```python
from build123d import *

# Parameters (mm, degrees)
SKETCH1_R           = 0.655
BOSS_EXTRUDE1_DEPTH = 16
CUT_EXTRUDE1_START  = -1.25
CUT_EXTRUDE1_DEPTH  = 1.25
SKETCH3_W           = 0.6
SKETCH3_H           = 0.3


with BuildPart() as part:
    # Sketch1 → Boss-Extrude1 (new body)
    with BuildSketch(Plane(origin=(0, 0, 0), x_dir=(1, 0, 0), z_dir=(0, 1, 0))):
        with Locations(Location((0, 0, 0), (0, 0, 270))):
            Circle(SKETCH1_R)
    extrude(amount=BOSS_EXTRUDE1_DEPTH)

    # Sketch2 → Cut-Extrude1 (cut)
    with BuildSketch(Plane(origin=(0, 16, 0), x_dir=(1, 0, 0), z_dir=(0, 1, 0)).offset(CUT_EXTRUDE1_START)):
        with BuildLine():
            Line((0, -0.655), (0, 0.655))
            ThreePointArc((0, 0.655), (0.655, 0), (0, -0.655))
        make_face()
    extrude(amount=CUT_EXTRUDE1_DEPTH, mode=Mode.SUBTRACT)

    # Sketch3 → Revolve1 (revolve)
    with BuildSketch(Plane.XY, mode=Mode.PRIVATE) as revolve1_sk:
        with Locations((0.655, 12)):
            Rectangle(SKETCH3_W, SKETCH3_H)
        with Locations((0.655, 10.7)):
            Rectangle(SKETCH3_W, SKETCH3_H)
    revolve(revolve1_sk.sketch.rotate(Axis((0, 16, 0), (0, -1, 0)), 90), axis=Axis((0, 16, 0), (0, -1, 0)))


solid = part.part
```
The listing builds one solid part. Answer for the finished solid, in the listing's coordinates (mm). A direction names the side the tool comes from. Round coordinates to 2 decimals unless told otherwise and drop trailing zeros. Order: outer loops, then holes, each group sorted by start corner. A loop starts at its lowest first (then second) coordinate and runs counter-clockwise, first axis right, second up. Notation, with made-up numbers: (-21, 27) -> (12, 27) arc R17 ccw to (12, 44) -> close; hole circle Ø2 at (89.5, -4.75). An arc over 180 degrees is marked (long way). Answer as CSV lines item,"result".
Q1. For a pull along Y with two mould halves and no side action, classify faces 1 (the flat face through (0, 0, 0)), 2 (the cylindrical face through (0.65, 11.34, -0.09)), 3 (the cylindrical face through (0.93, 10.7, -0.21)) as +Y half, -Y half, draft (parallel to the pull), parting line (faces both ways), or undercut.
Computed values:
face 1,"-Y half"
face 2,"undercut"
face 3,"draft"
Q2. A cutting plane is placed at C-C on y = 15. Determine the outline of the cut face in (x, z) (3 decimals).
Computed values:
outline,"(0, -0.655) -> (0, 0.655) arc R0.655 ccw to start"
Q3. A cutting plane is placed at B-B on y = 6.75. Determine the outline of the cut face in (x, z) (3 decimals).
Computed values:
outline,"circle Ø1.31 at (0, 0)"
Q4. A cutting plane is placed at A-A on z = 0. Determine the outline of the cut face in (x, y) (3 decimals).
Computed values:
outline,"(-0.955, 10.55) -> (-0.655, 10.55) -> (-0.655, 0) -> (0.655, 0) -> (0.655, 10.55) -> (0.955, 10.55) -> (0.955, 10.85) -> (0.655, 10.85) -> (0.655, 11.85) -> (0.955, 11.85) -> (0.955, 12.15) -> (0.655, 12.15) -> (0.655, 14.75) -> (0, 14.75) -> (0, 16) -> (-0.655, 16) -> (-0.655, 12.15) -> (-0.955, 12.15) -> (-0.955, 11.85) -> (-0.655, 11.85) -> (-0.655, 10.85) -> (-0.955, 10.85) -> close"
Q5. Given pin 1 (0.6 mm diameter, centred on y = 15, z = 0, fed in from +X) (3 decimals), flat-ended and moving along its own axis, determine where the tip first touches the part or whether it passes through.
Computed values:
pin 1,"stops at x = 0.655"
Q6. Consider line 1 (Y direction, x = -0.8, z = -0.3); line 2 (Z direction, x = 0.05, y = 1.25); line 3 (Y direction, x = 0.5, z = 0.3). Determine where each line is inside the solid, lowest interval first. Write a range as from..to.
Computed values:
line 1,"y = 10.55..10.85, 11.85..12.15"
line 2,"z = -0.65..0.65"
line 3,"y = 0..14.75"
Q7. Which of the six approach directions +Z, -Z, +X, -X, +Y, -Y give full straight-line access (tool end or side, diameter ignored) to faces 4 (the cylindrical face through (0.65, 5.2, -0.09)), 5 (the cylindrical face through (-0.581, 13.62, 0.302)), 6 (the cylindrical face through (0.93, 12, -0.21)), 7 (the flat face through (0, 15, 0))?
Computed values:
face 4,"-Y"
face 5,"+Y"
face 6,"+Y, -Y"
face 7,"+Z, -Z, +X, +Y"
